Geometry check sheet. Reference: the model listing, model coordinates, mm. A direction names the side the tool comes from. Round coordinates to 2 decimals unless told otherwise and drop trailing zeros. Order: outer loops, then holes, each group sorted by start corner. A loop starts at its lowest first (then second) coordinate and runs counter-clockwise, first axis right, second up.
(1) Go/stop test with flat-tipped pins: pin 1 (4 mm diameter, centred on y = 3.5, z = -10, fed in from +X); pin 2 (10 mm diameter, centred on x = -22.5, z = -7.5, fed in from -Y); pin 3 (4 mm diameter, centred on y = 3.5, z = -13.5, fed in from +X); pin 4 (3.5 mm diameter, centred on x = -22, z = -8, fed in from -Y). Record where each tip stops, or that it passes through.
(2) Release check for a two-part mould opening along X. For faces 5 (the face through (19.5, 6, -7.6)), 6 (the face through (-34.56, 4.06, -5.98)), 7 (the face through (0, 4, 0)) record: +X half, -X half, draft (parallel to the pull), parting line (faces both ways), or undercut.
(3) Set-up check for faces 1 (the face through (0, 0, -4)), 2 (the face through (-28.594, 1.972, -7.232)), 3 (the face through (15, 4, -12)), 4 (the face through (-17.42, 7.01, -5.39)): record each of +Z, -Z, +X, -X, +Y, -Y from which the full face is reachable in a straight line by a thin tool's end or side.
(4) Sectioned sample at B-B (y = 5). Give the number of separate pieces and of enclosed holes in the cut face, plus the area to 3 significant figures.
(5) Sectioned sample at A-A (x = -22.5). Record the boundary of the cut face in (y, z).
(6) Sectioned sample at D-D (x = 8.5). Record the boundary of the cut face in (y, z).
(7) Material ranges on line 1 along X through (y, z) = (2, -10.5); line 2 along Z through (x, y) = (-22.5, 7.05); line 3 along X through (y, z) = (5.5, -9.5), recorded low to high.
from build123d import *

# Parameters (mm, degrees)
ESQUISSE1_R             = 3
BOSS_EXTRU_1_DEPTH      = 8
ESQUISSE3_R             = 5.5
ESQUISSE3_R_2           = 4.5
ENL_V_MAT_EXTRU_2_DEPTH = 2
ESQUISSE4_R             = 6.1
ENL_V_MAT_EXTRU_3_DEPTH = 4
CONG_1_R                = 5
CONG_2_R                = 3
CONG_3_R                = 4


with BuildPart() as part:
    # Esquisse1 → Boss.-Extru.1 (new body)
    with BuildSketch(Plane(origin=(0, 0, 0), x_dir=(1, 0, 0), z_dir=(0, 1, 0))):
        Polygon((-35, 0), (35, 0), (35, 6), (20, 21), (15, 21), (15, 5), (-15, 5), (-15, 21), (-20, 21), (-35, 6), align=None)
        with Locations((22.5, 7.5)):
            Circle(ESQUISSE1_R, mode=Mode.SUBTRACT)
        with Locations((-22.5, 7.5)):
            Circle(ESQUISSE1_R, mode=Mode.SUBTRACT)
    extrude(amount=BOSS_EXTRU_1_DEPTH)

    # Esquisse3 → Enlèv. mat.-Extru.2 (cut)
    with BuildSketch(Plane(origin=(0, 8, 0), x_dir=(1, 0, 0), z_dir=(0, 1, 0))):
        with Locations((-22.5, 7.5)):
            Circle(ESQUISSE3_R)
        with Locations((-22.5, 7.5)):
            Circle(ESQUISSE3_R_2, mode=Mode.SUBTRACT)
        with Locations((22.5, 7.5)):
            Circle(ESQUISSE3_R)
        with Locations((22.5, 7.5)):
            Circle(ESQUISSE3_R_2, mode=Mode.SUBTRACT)
    extrude(amount=-ENL_V_MAT_EXTRU_2_DEPTH, mode=Mode.SUBTRACT)

    # Esquisse4 → Enlèv. mat.-Extru.3 (cut)
    with BuildSketch(Plane.XZ):
        with Locations((-22.5, -7.5)):
            Circle(ESQUISSE4_R)
        with Locations((22.5, -7.5)):
            Circle(ESQUISSE4_R)
    extrude(amount=-ENL_V_MAT_EXTRU_3_DEPTH, mode=Mode.SUBTRACT)

    # Congé1
    cong_1_edges = [part.edges().sort_by_distance(p)[0] for p in [
        (-35, 4, -6),
        (-20, 4, -21),
        (20, 4, -21),
        (35, 4, -6),
    ]]
    fillet(cong_1_edges, radius=CONG_1_R)

    # Congé2
    cong_2_edges = [part.edges().sort_by_distance(p)[0] for p in [
        (15, 4, -21),
        (-15, 4, -21),
    ]]
    fillet(cong_2_edges, radius=CONG_2_R)

    # Congé3
    cong_3_edges = [part.edges().sort_by_distance(p)[0] for p in [
        (35, 4, 0),
        (-35, 4, 0),
    ]]
    fillet(cong_3_edges, radius=CONG_3_R)


solid = part.part
Answer below:
1. pin 1: stops at x = 33
1. pin 2: stops at y = 4
1. pin 3: stops at x = 29.5
1. pin 4: passes through
2. face 5: undercut
2. face 6: -X half
2. face 7: draft
3. face 1: +Z, -Z, +X, -X, -Y
3. face 2: -Y
3. face 3: -Z, +Y, -Y
3. face 4: +Y
4. separate pieces: 1
4. enclosed holes: 2
4. area: 696 mm2
5. outline: (0, -18.5) - (8, -18.5) - (8, -13) - (6, -13) - (6, -12) - (8, -12) - (8, -10.5) - (4, -10.5) - (4, -13.6) - (0, -13.6) - close; (0, -1.4) - (4, -1.4) - (4, -4.5) - (8, -4.5) - (8, -3) - (6, -3) - (6, -2) - (8, -2) - (8, 0) - (0, 0) - close
6. outline: (0, -5) - (8, -5) - (8, 0) - (0, 0) - close
7. line 1: x = -30.5 to -27.81, -17.19 to -15, 15 to 17.19, 27.81 to 30.5
7. line 2: z = -18.5 to -13, -12 to -10.5, -4.5 to -3, -2 to 0
7. line 3: x = -31.5 to -24.74, -20.26 to -15, 15 to 20.26, 24.74 to 31.5
